The listing builds one solid part. Answer for the finished solid, in the listing's coordinates (mm). A direction names the side the tool comes from. Give positions to 0.01 mm unless a question says otherwise; leave off trailing zeros. Loops run counter-clockwise (first coordinate to the right, second up) from the corner with the lowest first, then second, coordinate; pieces in that order, holes last.
Item 1: The mould has two halves that part along Z. Classify faces 4 (the face through (12, 0, 0)), 5 (the face through (1, 2, 0)), 6 (the face through (0.49, 0.86, 0.51)): pulls with the +Z half, pulls with the -Z half, needs draft (parallel to the pull), parting line crosses it, or undercut.
Item 2: A tool of negligible diameter and unlimited length cuts with its end or side. For faces 1 (the face through (0, 0, -1.3)), 2 (the face through (6.82, -0.45, 1.43)), 3 (the face through (0.49, -0.87, 0.49)), from which of +Z, -Z, +X, -X, +Y, -Y can it reach the whole face along a straight path? Write none if from no direction.
Item 3: Section B-B, the plane x = 7.25 is taken. Give the vertices of the cut face in (y, z).
Item 4: Section A-A, the plane y = 0 is taken. Give the vertices of the cut face in (x, z), and give its area (4 significant figures).
Item 5: Consider line 1 along Z through (x, y) = (3.5, -0.1); line 2 along X through (y, z) = (1.05, 0). Determine where each line is inside the solid, lowest interval first.
Item 6: Each of these flat-tipped pins is pushed along its axis until it touches: pin 1 Ø2 at (x, z) = (2.5, -1.5) entering from +Y; pin 2 Ø2 at (x, y) = (4.5, -2) entering from +Z; pin 3 Ø0.8 at (x, y) = (0.5, 0) entering from -Z. Where does it stop, or does it pass through?
from build123d import *

# Parameters (mm, degrees)
CUT_EXTRUDE_1_DEPTH = 1


with BuildPart() as part:
    # 草图1 → 旋转1 (revolve)
    with BuildSketch(Plane.XY, mode=Mode.PRIVATE) as revolve_1_sk:
        Polygon((0, 0), (0, 3), (1.5, 1.5), (12, 1.5), (12, 0), align=None)
    revolve(revolve_1_sk.sketch.rotate(Axis((0, 0, 0), (1, 0, 0)), 90), axis=Axis((0, 0, 0), (1, 0, 0)))

    # 草图2 → 切除-拉伸1 (cut)
    with BuildSketch(Plane.ZY):
        Polygon((0, 1.154700538), (-1, 0.577350269), (-1, -0.577350269), (0, -1.154700538), (1, -0.577350269), (1, 0.577350269), align=None)
    extrude(amount=-CUT_EXTRUDE_1_DEPTH, mode=Mode.SUBTRACT)


solid = part.part
Worked answers:
1. face 4: needs draft
1. face 5: parting line crosses it
1. face 6: undercut
2. face 1: +Z, -Z, -X, +Y, -Y
2. face 2: +X
2. face 3: -X
3. outline: circle Ø3 at (0, 0)
4. outline: (0, -3) - (1.5, -1.5) - (12, -1.5) - (12, 1.5) - (1.5, 1.5) - (0, 3) - (0, 1) - (1, 1) - (1, -1) - (0, -1) - close
4. area: 36.25 mm2
5. line 1: z = -1.5 to 1.5
5. line 2: x = 1 to 12
6. pin 1: stops at y = 1.41
6. pin 2: stops at z = 1.12
6. pin 3: stops at z = -2.9
